from build123d import *

# Parameters (mm, degrees)
SKETCH2_W               = 150
SKETCH2_H               = 1040
BOSS_EXTRUDE1_DEPTH     = 20
SKETCH3_W               = 150
SKETCH3_H               = 20
BOSS_EXTRUDE2_DEPTH     = 150
CUT_EXTRUDE1_DEPTH      = 1054.434857977
CUT_EXTRUDE1_DEPTH_BACK = 1054.434857977
SKETCH4_W               = 25
SKETCH4_H               = 25
SKETCH5_R               = 6
BOSS_EXTRUDE3_DEPTH     = 10
CUT_EXTRUDE2_REACH      = 1055.435
SKETCH6_W               = 150
SKETCH6_H               = 41


with BuildPart() as part:
    # Sketch2 → Boss-Extrude1 (new body)
    with BuildSketch(Plane(origin=(0, 0, 0), x_dir=(1, 0, 0), z_dir=(0, 1, 0))):
        Rectangle(SKETCH2_W, SKETCH2_H)
    extrude(amount=-BOSS_EXTRUDE1_DEPTH)

    # Sketch3 → Boss-Extrude2 (add)
    with BuildSketch(Plane(origin=(0, 0, 0), x_dir=(1, 0, 0), z_dir=(0, 1, 0))):
        with Locations((0, -510)):
            Rectangle(SKETCH3_W, SKETCH3_H)
        with Locations((0, 510)):
            Rectangle(SKETCH3_W, SKETCH3_H)
    extrude(amount=BOSS_EXTRUDE2_DEPTH)

    # Sketch4 → Cut-Extrude1 (cut, two sides: drawn at the far end of the back side and taken through both)
    with BuildSketch(Plane.XY.offset(520).offset(-CUT_EXTRUDE1_DEPTH_BACK)):
        with Locations((0, 75)):
            Rectangle(SKETCH4_W, SKETCH4_H)
    extrude(amount=CUT_EXTRUDE1_DEPTH + CUT_EXTRUDE1_DEPTH_BACK, mode=Mode.SUBTRACT)

    # Sketch5 → Boss-Extrude3 (add)
    with BuildSketch(Plane.XZ.offset(20)):
        with Locations(Location((-55, 500, 0), (0, 0, 270))):
            Circle(SKETCH5_R)
        with Locations(Location((55, 500, 0), (0, 0, 270))):
            Circle(SKETCH5_R)
        with Locations(Location((-55, -500, 0), (0, 0, 270))):
            Circle(SKETCH5_R)
        with Locations(Location((55, -500, 0), (0, 0, 270))):
            Circle(SKETCH5_R)
    extrude(amount=BOSS_EXTRUDE3_DEPTH)

    # Sketch6 → Cut-Extrude2 (cut, up to next)
    with BuildSketch(Plane.XY.offset(520), mode=Mode.PRIVATE) as cut_extrude2_sk1:
        with Locations((0, 129.5)):
            Rectangle(SKETCH6_W, SKETCH6_H)
    cut_extrude2_tool1 = extrude(cut_extrude2_sk1.sketch, amount=-CUT_EXTRUDE2_REACH, mode=Mode.PRIVATE) & part.part
    add(cut_extrude2_tool1.solids().sort_by_distance((0, 129.5, 520))[0], mode=Mode.SUBTRACT)


solid = part.part
Geometry: final body of the model. Coordinates: model frame, mm. A direction names the side the tool comes from. Give positions to 0.01 mm unless a question says otherwise; leave off trailing zeros. Loops run counter-clockwise (first coordinate to the right, second up) from the corner with the lowest first, then second, coordinate; pieces in that order, holes last. Notation, with made-up numbers: (57, 47) -> (63, 47) arc R12 cw to (63, 62) -> close; hole circle Ø6 at (10.25, 74). An arc over 180 degrees is marked (long way). Put each result on its own line as item: value.
1. Cut plane A-A (y = 15). Return the cut outline in (x, z), plus the area to 3 significant figures.
Taken from the geometry:
outline: (-75, -520) -> (75, -520) -> (75, -500) -> (-75, -500) -> close; (-75, 500) -> (75, 500) -> (75, 520) -> (-75, 520) -> close
area: 6,000 mm2
2. Set-up query: faces 1 (the flat face through (-1, 0, -7)), 2 (the flat face through (12.5, 75, -510)), 3 (the flat face through (-1, 109, 510)). Return all of +Z, -Z, +X, -X, +Y, -Y with unobstructed straight access to the full face (end or side cutting, diameter ignored); none if empty.
Taken from the geometry:
face 1: +X, -X, +Y
face 2: +Z, -Z
face 3: +Z, +X, -X, +Y
3. Ray query, line 1 along Z through (x, y) = (-33.5, 21); line 2 along Y through (x, z) = (-6, -193); line 3 along Z through (x, y) = (-35, 128.5). Return the intervals inside material, ascending. Write a range as [from, to].
Taken from the geometry:
line 1: z = [-520, -500], [500, 520]
line 2: y = [-20, 0]
line 3: z = [-520, -500]
4. Cut plane C-C (z = 451). Return the cut outline in (x, y), plus the area to 3 significant figures.
Taken from the geometry:
outline: (-75, -20) -> (75, -20) -> (75, 0) -> (-75, 0) -> close
area: 3,000 mm2
5. Pin query (flat end, axial travel): P1, Ø1, axis at x = 15.5, z = 165, coming from the -Y side; P2, Ø6, axis at x = 6, z = 511.5, coming from the +Y side. Return the tip coordinate at first contact, or that it passes through.
Taken from the geometry:
P1: stops at y = -20
P2: stops at y = 109
6. Cut plane B-B (x = -30). Return the cut outline in (y, z), plus the area to 3 significant figures.
Taken from the geometry:
outline: (-20, -520) -> (150, -520) -> (150, -500) -> (0, -500) -> (0, 500) -> (109, 500) -> (109, 520) -> (-20, 520) -> close
area: 26,000 mm2
7. Pull-direction query (X, two-part tool) for faces 4 (the flat face through (0, 87.5, -510)), 5 (the flat face through (-18, 66, -520)), 6 (the flat face through (75, -5, 79)); classes: released by +X, released by -X, zero draft, split by the parting line, or undercut.
Taken from the geometry:
face 4: undercut
face 5: zero draft
face 6: released by +X
